from build123d import *

# Parameters (mm, degrees)
SKETCH1_R           = 2.5
SKETCH1_R_2         = 1.5
BOSS_EXTRUDE1_DEPTH = 3


with BuildPart() as part:
    # Sketch1 → Boss-Extrude1 (new body)
    with BuildSketch(Plane.XY):
        with BuildLine():
            Line((-19, 0), (-19, -32))
            Line((-19, -32), (-14.8, -32))
            Line((-14.8, -32), (-14.8, -45))
            Line((-14.8, -45), (-5, -45))
            Line((-5, -45), (-5, -42))
            Line((-5, -42), (5, -42))
            Line((5, -42), (5, -45))
            Line((5, -45), (19, -45))
            Line((19, -45), (19, 0))
            ThreePointArc((19, 0), (0, 19), (-19, 0))
        make_face()
        Circle(SKETCH1_R, mode=Mode.SUBTRACT)
        with Locations((-14, -27)):
            Circle(SKETCH1_R_2, mode=Mode.SUBTRACT)
        with Locations(Location((14, -27, 0), (0, 0, 180))):
            Circle(SKETCH1_R_2, mode=Mode.SUBTRACT)
    extrude(amount=BOSS_EXTRUDE1_DEPTH)


solid = part.part
Geometry check sheet. Reference: the model listing, model coordinates, mm. A direction names the side the tool comes from. Round coordinates to 2 decimals unless told otherwise and drop trailing zeros. Order: outer loops, then holes, each group sorted by start corner. A loop starts at its lowest first (then second) coordinate and runs counter-clockwise, first axis right, second up. Notation, with made-up numbers: M 89,-11 L 137,-11 A19 ccw 137,26 Z; hole C -37.5,6.25 d7. An arc over 180 degrees is marked long. Answer in a Markdown table with one row per item.
(1) Sectioned sample at B-B, the plane x = 0. Record the cut outline in (y, z).
Responses:
| item | result |
|---|---|
| outline | M -42,0 L -2.5,0 L -2.5,3 L -42,3 Z; M 2.5,0 L 19,0 L 19,3 L 2.5,3 Z |
(2) Sectioned sample at C-C, the plane z = 1.3. Record the cut outline in (x, y).
Responses:
| item | result |
|---|---|
| outline | M -19,-32 L -14.8,-32 L -14.8,-45 L -5,-45 L -5,-42 L 5,-42 L 5,-45 L 19,-45 L 19,0 A19 ccw -19,0 Z; hole C -14,-27 d3; hole C 0,0 d5; hole C 14,-27 d3 |
(3) Tool access check on faces 1 (the face through (-10, -45, 1)), 2 (the face through (5, -43, 1)), 3 (the face through (-17, -32, 1)). Record the directions out of +Z, -Z, +X, -X, +Y, -Y that give a thin tool (end or side, any length) a straight path to the whole face; none if there is none.
Responses:
| item | result |
|---|---|
| face 1 | +Z, -Z, +X, -X, -Y |
| face 2 | +Z, -Z, -Y |
| face 3 | +Z, -Z, -X, -Y |
(4) Scan lines: probe 1 along Y at (x, z) = (0, 2.2); probe 2 along Y at (x, z) = (-14, 1.4); probe 3 along X at (y, z) = (-33, 0.7). Record each from-to range of solid material in increasing order. Write a range as from..to.
Responses:
| item | result |
|---|---|
| probe 1 | y = -42..-2.5, 2.5..19 |
| probe 2 | y = -45..-28.5, -25.5..12.85 |
| probe 3 | x = -14.8..19 |
(5) Sectioned sample at A-A, the plane y = -27. Record the cut outline in (x, z), and give its area (3 significant figures).
Responses:
| item | result |
|---|---|
| outline | M -19,0 L -15.5,0 L -15.5,3 L -19,3 Z; M -12.5,0 L 12.5,0 L 12.5,3 L -12.5,3 Z; M 15.5,0 L 19,0 L 19,3 L 15.5,3 Z |
| area | 96.0 mm² |
(6) Sectioned sample at D-D, the plane x = 14. Record the cut outline in (y, z).
Responses:
| item | result |
|---|---|
| outline | M -45,0 L -28.5,0 L -28.5,3 L -45,3 Z; M -25.5,0 L 12.85,0 L 12.85,3 L -25.5,3 Z |
(7) Draft check along Y on faces 4 (the face through (0, 19, 1)), 5 (the face through (14.195, -28.487, 1.479)), 6 (the face through (-19, -16, 1)). Enter one of: released by +Y, released by -Y, zero draft, split by the parting line, or undercut.
Responses:
| item | result |
|---|---|
| face 4 | released by +Y |
| face 5 | undercut |
| face 6 | zero draft |
(8) Go/stop test with flat-tipped pins: P1, Ø1.8, axis at x = -14, y = -27, coming from the -Z side; P2, Ø0.9, axis at x = -2, z = 2, coming from the -Y side; P3, Ø1, axis at y = 4.5, z = 1.5, coming from the +X side. Record where each tip stops, or that it passes through.
Responses:
| item | result |
|---|---|
| P1 | passes through |
| P2 | stops at y = -42 |
| P3 | stops at x = 18.57 |
